from build123d import *

# Parameters (mm, degrees)
SKETCH1_W           = 150
SKETCH1_H           = 150
BOSS_EXTRUDE1_DEPTH = 6
CUT_EXTRUDE2_DEPTH  = 6
SKETCH3_W           = 55
SKETCH3_H           = 200
BOSS_EXTRUDE3_DEPTH = 6
SKETCH4_W           = 160
SKETCH4_H           = 55
BOSS_EXTRUDE4_DEPTH = 6
SKETCH5_W           = 55
SKETCH5_H           = 200
BOSS_EXTRUDE5_DEPTH = 6
SKETCH6_W           = 160
SKETCH6_H           = 55
BOSS_EXTRUDE6_DEPTH = 6


with BuildPart() as part:
    # Sketch1 → Boss-Extrude1 (new body)
    with BuildSketch(Plane(origin=(0, 0, 0), x_dir=(1, 0, 0), z_dir=(0, 1, 0))):
        Rectangle(SKETCH1_W, SKETCH1_H)
    extrude(amount=BOSS_EXTRUDE1_DEPTH)

    # Sketch2 → Cut-Extrude2 (cut)
    with BuildSketch(Plane(origin=(0, 6, 0), x_dir=(1, 0, 0), z_dir=(0, 1, 0))):
        Polygon((-5, -65), (-5, -5), (-65, -65), align=None)
        Polygon((-10, 0), (-5, 5), (-15, 5), align=None)
        Polygon((-5, 65), (-65, 65), (-5, 5), align=None)
        Polygon((-65, 5), (-15, 5), (-65, 55), align=None)
        Polygon((-10, 0), (-15, 5), (-65, 5), (-65, -5), (-15, -5), align=None)
        Polygon((-5, -5), (-10, 0), (-15, -5), align=None)
        Polygon((-65, -55), (-15, -5), (-65, -5), align=None)
        Polygon((5, 5), (65, 65), (5, 65), align=None)
        Polygon((65, -65), (5, -5), (5, -65), align=None)
        Polygon((15, 5), (5, 5), (10, 0), align=None)
        Polygon((65, 5), (15, 5), (10, 0), (15, -5), (65, -5), align=None)
        Polygon((65, 55), (15, 5), (65, 5), align=None)
        Polygon((15, -5), (10, 0), (5, -5), align=None)
        Polygon((65, -5), (15, -5), (65, -55), align=None)
    extrude(amount=-CUT_EXTRUDE2_DEPTH, mode=Mode.SUBTRACT)

    # Sketch3 → Boss-Extrude3 (add)
    with BuildSketch(Plane(origin=(0, 6, 0), x_dir=(1, 0, 0), z_dir=(0, 1, 0))):
        with Locations((102.5, -25)):
            Rectangle(SKETCH3_W, SKETCH3_H)
        Polygon((65, -65), (5, -5), (5, -65), align=None)
        Polygon((10, 0), (5, -5), (15, -5), (65, -55), (65, 55), (15, 5), (5, 5), align=None)
        Polygon((5, 65), (5, 5), (65, 65), align=None)
        Polygon((-5, -65), (-5, -5), (-65, -65), align=None)
        Polygon((-15, -5), (-5, -5), (-10, 0), (-5, 5), (-15, 5), (-65, 55), (-65, -55), align=None)
        Polygon((-65, 65), (-5, 5), (-5, 65), align=None)
    extrude(amount=-BOSS_EXTRUDE3_DEPTH)

    # Sketch4 → Boss-Extrude4 (add)
    with BuildSketch(Plane(origin=(0, 6, 0), x_dir=(1, 0, 0), z_dir=(0, 1, 0))):
        with Locations((0, -102.5)):
            Rectangle(SKETCH4_W, SKETCH4_H)
    extrude(amount=-BOSS_EXTRUDE4_DEPTH)

    # Sketch5 → Boss-Extrude5 (add)
    with BuildSketch(Plane(origin=(0, 6, 0), x_dir=(1, 0, 0), z_dir=(0, 1, 0))):
        with Locations((-102.5, 25)):
            Rectangle(SKETCH5_W, SKETCH5_H)
    extrude(amount=-BOSS_EXTRUDE5_DEPTH)

    # Sketch6 → Boss-Extrude6 (add)
    with BuildSketch(Plane(origin=(0, 6, 0), x_dir=(1, 0, 0), z_dir=(0, 1, 0))):
        with Locations((-5, 102.5)):
            Rectangle(SKETCH6_W, SKETCH6_H)
    extrude(amount=-BOSS_EXTRUDE6_DEPTH)


solid = part.part
The listing builds one solid part. Answer for the finished solid, in the listing's coordinates (mm). A direction names the side the tool comes from. Round coordinates to 2 decimals unless told otherwise and drop trailing zeros. Write each loop counter-clockwise with the first axis right and the second up, starting at its lowest first coordinate (ties: lowest second). Pieces come first, ordered by that corner, then holes. Notation, with made-up numbers: M 76,9 L 103,9 A28 ccw 103,27 Z; hole C -22,77 d6. An arc over 180 degrees is marked long. Write each question's results on one line, items separated by ' | '. Start each with the question number.
(1) Find the intervals of material crossed by line 1 (X direction, y = 1.85, z = -98); line 2 (Z direction, x = 75.5, y = 3.9); line 3 (Z direction, x = -96, y = 4.8), in increasing order.
(2) The part is cut by section B-B, the plane z = -78. Write down the section's boundary in (x, y).
(3) Each of these flat-tipped pins is pushed along its axis until it touches: P1, Ø1.5, axis at y = 3, z = 127, coming from the +X side; P2, Ø1.8, axis at y = 1.5, z = -115, coming from the +X side; P3, Ø1.8, axis at x = -100.5, y = 3.5, coming from the +Z side. Where does it stop, or does it pass through?
(4) The part is cut by section A-A, the plane y = 0.9. Write down the section's boundary in (x, z).
(5) For faces 1 (the flat face through (105, 3, 125)), 2 (the flat face through (102, 3, -75)), 3 (the flat face through (-80, 3, 103)), 4 (the flat face through (-108, 3, -125)), determine the directions among +Z, -Z, +X, -X, +Y, -Y from which every point of the face is accessible in a straight line to the end or side of a thin tool.
(6) The part is cut by section C-C, the plane x = 85. Write down the section's boundary in (y, z).
Worked answers:
1) line 1: x = -130 to 75 | line 2: z = -75 to 130 | line 3: z = -125 to 75
2) outline: M -130,0 L 75,0 L 75,6 L -130,6 Z
3) P1: stops at x = 80 | P2: stops at x = 75 | P3: stops at z = 75
4) outline: M -130,-125 L -85,-125 L -85,-130 L 75,-130 L 75,-75 L 130,-75 L 130,125 L 80,125 L 80,130 L -80,130 L -80,75 L -130,75 Z
5) face 1: +Z, +X, +Y, -Y | face 2: -Z, +X, +Y, -Y | face 3: +Z, -X, +Y, -Y | face 4: -Z, -X, +Y, -Y
6) outline: M 0,-75 L 6,-75 L 6,125 L 0,125 Z
